Design review of the part shown in the three views and the two pictorial views. Dimensions are in mm from the part's minimum x, y and z. A direction names the side the tool comes from. Give positions to 0.01 mm unless a question says otherwise; leave off trailing zeros. Write each loop counter-clockwise with the first axis right and the second up, starting at its lowest first coordinate (ties: lowest second). Pieces come first, ordered by that corner, then holes.
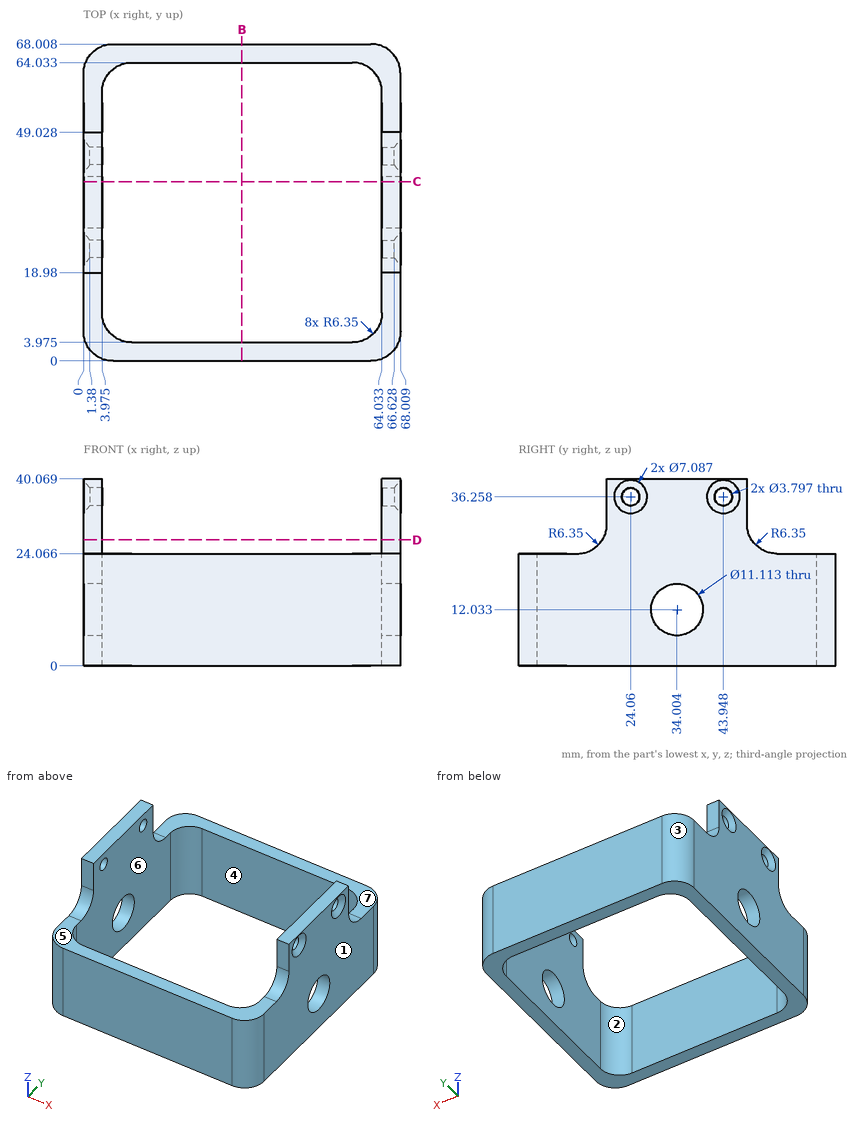
(1) Tool access review of the marked faces 5, 6 and 7: name each direction out of +Z, -Z, +X, -X, +Y, -Y from which nothing blocks a thin tool from reaching the whole face with its end or side.
Resolved:
face 5: +Z, +X, -X, -Y
face 6: +Z, -Z
face 7: +Z, +X, -X, +Y
(2) Mouldability with a two-part tool opening along X and no side actions: class the marked faces 1, 2, 3 and 4 as pulls with the +X half, pulls with the -X half, needs draft (parallel to the pull), parting line crosses it, or undercut.
Resolved:
face 1: pulls with the +X half
face 2: undercut
face 3: pulls with the -X half
face 4: undercut
(3) Consider section D-D, the plane z = 27. Give the boundary of the cut face in (x, y) (1 decimal).
Resolved:
outline: (0, 18) - (4, 18) - (4, 50) - (0, 50) - close; (64, 18) - (68, 18) - (68, 50) - (64, 50) - close
(4) Clearance check with flat-ended pins moving along their axes: P1, Ø4.5, axis at x = 66.5, z = 34, coming from the -Y side; P2, Ø1.2, axis at x = 65, z = 35.5, coming from the +Y side; P3, Ø10, axis at x = 40.5, y = 3.5, coming from the +Z side. State where each tip first meets the part, or that it passes through.
Resolved:
P1: stops at y = 18.98
P2: stops at y = 49.03
P3: stops at z = 24.07
(5) Consider section C-C, the plane y = 38.5. Give the boundary of the cut face in (x, z) (1 decimal).
Resolved:
outline: (0, 0) - (4, 0) - (4, 8.8) - (0, 8.8) - close; (0, 15.3) - (4, 15.3) - (4, 40.1) - (0, 40.1) - close; (64, 0) - (68, 0) - (68, 8.8) - (64, 8.8) - close; (64, 15.3) - (68, 15.3) - (68, 40.1) - (64, 40.1) - close
(6) Consider section B-B, the plane x = 34. Give the boundary of the cut face in (y, z) (1 decimal), then the cut area to 3 significant figures.
Resolved:
outline: (0, 0) - (4, 0) - (4, 24.1) - (0, 24.1) - close; (64, 0) - (68, 0) - (68, 24.1) - (64, 24.1) - close
area: 191 mm2
(7) To check wall thickness, follow L1, parallel to Y at x = 34.5, z = 4.5 (1 decimal); L2, parallel to Z at x = 41.5, y = 65.5. State the ranges of each line that lie inside material, in increasing order.
Resolved:
L1: y = 0 to 4, 64 to 68
L2: z = 0 to 24.07
